```python
from build123d import *

# Parameters (mm, degrees)
SKETCH1_R           = 4.2545
SKETCH1_R_2         = 3.175
BOSS_EXTRUDE1_DEPTH = 11.303
SKETCH2_R           = 3.175
BOSS_EXTRUDE2_DEPTH = 15.1257
SKETCH5_W           = 5.9817
SKETCH5_H           = 3.048
CUT_EXTRUDE2_DEPTH  = 15.1257


with BuildPart() as part:
    # Sketch1 → Boss-Extrude1 (new, symmetric)
    with BuildSketch(Plane.XY):
        with Locations(Location((0, 0, 0), (0, 0, 180))):
            Circle(SKETCH1_R)
        with Locations(Location((0, 0, 0), (0, 0, 180))):
            Circle(SKETCH1_R_2, mode=Mode.SUBTRACT)
    extrude(amount=BOSS_EXTRUDE1_DEPTH, both=True)

    # Sketch2 → Boss-Extrude2 (add, symmetric)
    with BuildSketch(Plane.XY):
        with Locations(Location((0, 0, 0), (0, 0, 180))):
            Circle(SKETCH2_R)
    extrude(amount=BOSS_EXTRUDE2_DEPTH, both=True)

    # Sketch5 → Cut-Extrude2 (cut, symmetric)
    with BuildSketch(Plane(origin=(0, 0, 0), x_dir=(0, 0, -1), z_dir=(1, 0, 0))):
        with Locations((-2.99085, 0)):
            Rectangle(SKETCH5_W, SKETCH5_H)
        with Locations((2.99085, 0)):
            Rectangle(SKETCH5_W, SKETCH5_H)
    extrude(amount=CUT_EXTRUDE2_DEPTH, both=True, mode=Mode.SUBTRACT)


solid = part.part
```
Check sheet for the modelled part. Datum: model origin and axes. Units: mm. A direction names the side the tool comes from. Give positions to 0.01 mm unless a question says otherwise; leave off trailing zeros. Order: outer loops, then holes, each group sorted by start corner. A loop starts at its lowest first (then second) coordinate and runs counter-clockwise, first axis right, second up. Notation, with made-up numbers: (33, -26.75) -> (52, -26.75) arc R17 ccw to (52, -3.75) -> close; hole circle Ø1 at (38, 64). An arc over 180 degrees is marked (long way). Use CSV: the item, a comma, the result in double quotes. Start each with the question number.
1) Material ranges on line 1 (Z direction, x = 2.25, y = -1.25); line 2 (Z direction, x = -3.25, y = -0.25); line 3 (Y direction, x = 2, z = -2), recorded low to high. Write a range as from..to.
2) Set-up check for faces 1 (the face through (-1.5, 2.8, -13.2)), 2 (the face through (0, 0, 15.126)), 3 (the face through (0, 1.524, 0)): record each of +Z, -Z, +X, -X, +Y, -Y from which the full face is reachable in a straight line by a thin tool's end or side.
3) Sectioned sample at C-C, the plane z = 1. Record the boundary of the cut face in (x, y).
4) Sectioned sample at B-B, the plane x = 0. Record the boundary of the cut face in (y, z) (1 decimal).
5) Sectioned sample at A-A, the plane y = 0. Record the boundary of the cut face in (x, z) (1 decimal).
6) Go/stop test with flat-tipped pins: P1, Ø3, axis at y = -3, z = -3.5, coming from the +X side; P2, Ø3, axis at x = 2, z = -5, coming from the -Y side (3 decimals). Record where each tip stops, or that it passes through.
7) Sectioned sample at D-D, the plane x = 2.5. Record the boundary of the cut face in (y, z).
8) Mould release check, pull along Y, two halves, no side actions. Record for faces 4 (the face through (-1.5, 2.8, 13.2)), 5 (the face through (0, -1.524, 0)), 6 (the face through (2, 3, 11.303)): released by +Y, released by -Y, zero draft, split by the parting line, or undercut.
Recorded:
1,line 1,"-15.13..-5.98, 5.98..15.13"
1,line 2,"-11.3..-5.98, 5.98..11.3"
1,line 3,"-3.76..-1.52, 1.52..3.76"
2,face 1,"-Z"
2,face 2,"+Z, +X, -X, +Y, -Y"
2,face 3,"+X, -X"
3,outline,"(-3.97, -1.52) arc R4.25 ccw to (3.97, -1.52) -> close; (-3.97, 1.52) -> (3.97, 1.52) arc R4.25 ccw to start"
4,outline,"(-4.3, -11.3) -> (-3.2, -11.3) -> (-3.2, -15.1) -> (3.2, -15.1) -> (3.2, -11.3) -> (4.3, -11.3) -> (4.3, 11.3) -> (3.2, 11.3) -> (3.2, 15.1) -> (-3.2, 15.1) -> (-3.2, 11.3) -> (-4.3, 11.3) -> close; hole (-1.5, -6) -> (1.5, -6) -> (1.5, 6) -> (-1.5, 6) -> close"
5,outline,"(-4.3, -11.3) -> (-3.2, -11.3) -> (-3.2, -15.1) -> (3.2, -15.1) -> (3.2, -11.3) -> (4.3, -11.3) -> (4.3, -6) -> (-4.3, -6) -> close; (-4.3, 6) -> (4.3, 6) -> (4.3, 11.3) -> (3.2, 11.3) -> (3.2, 15.1) -> (-3.2, 15.1) -> (-3.2, 11.3) -> (-4.3, 11.3) -> close"
6,P1,"x = 3.97"
6,P2,"y = -4.225"
7,outline,"(-3.44, -11.3) -> (-1.96, -11.3) -> (-1.96, -15.13) -> (1.96, -15.13) -> (1.96, -11.3) -> (3.44, -11.3) -> (3.44, 11.3) -> (1.96, 11.3) -> (1.96, 15.13) -> (-1.96, 15.13) -> (-1.96, 11.3) -> (-3.44, 11.3) -> close; hole (-1.52, -5.98) -> (1.52, -5.98) -> (1.52, 5.98) -> (-1.52, 5.98) -> close"
8,face 4,"split by the parting line"
8,face 5,"undercut"
8,face 6,"zero draft"
